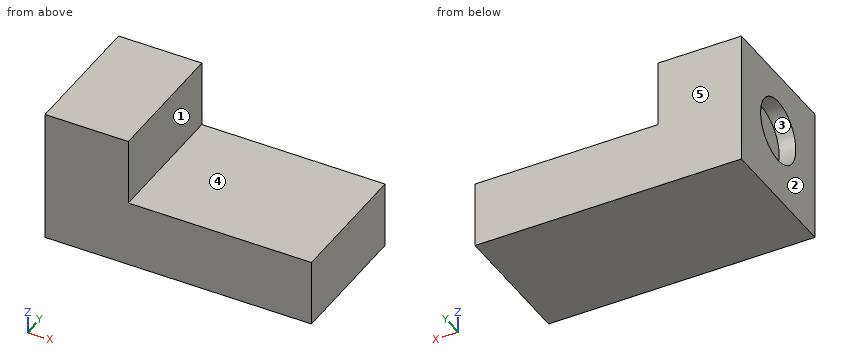
```python
from build123d import *

# Parameters (mm, degrees)
SKETCH_1_W          = 80
SKETCH_1_H          = 40
EXTRUDE_1_DEPTH     = 20
SKETCH_2_W          = 25
SKETCH_2_H          = 40
EXTRUDE_2_DEPTH     = 20
SKETCH_3_R          = 9.55930051
CUT_EXTRUDE_1_DEPTH = 5


with BuildPart() as part:
    # 草图1 → 凸台-拉伸1 (new body)
    with BuildSketch(Plane.XY):
        Rectangle(SKETCH_1_W, SKETCH_1_H)
    extrude(amount=EXTRUDE_1_DEPTH)

    # 草图2 → 凸台-拉伸2 (add)
    with BuildSketch(Plane.XY.offset(20)):
        with Locations((-27.5, 0)):
            Rectangle(SKETCH_2_W, SKETCH_2_H)
    extrude(amount=EXTRUDE_2_DEPTH)

    # 草图3 → 切除-拉伸1 (cut)
    with BuildSketch(Plane.ZY.offset(40)):
        with Locations((21.858234258, 0)):
            Circle(SKETCH_3_R)
    extrude(amount=-CUT_EXTRUDE_1_DEPTH, mode=Mode.SUBTRACT)


solid = part.part
```
Source: CAD feature listing. Evaluate the final solid. Frame: model axes, mm. Face numbers are marked on the shaded views. A direction names the side the tool comes from. Coordinates: 2 decimals unless noted, no trailing zeros. Loops run counter-clockwise (first coordinate to the right, second up) from the corner with the lowest first, then second, coordinate; pieces in that order, holes last. Notation, with made-up numbers: (33.5, 22.5) - (45.5, 22.5) arc R29 ccw to (45.5, 53.5) - close; hole circle Ø6 at (-17.5, -20.75). An arc over 180 degrees is marked (long way). Answer as CSV lines item,"result".
1. Section A-A (y = 0). Return loops of the section in (x, z), then the cut area to 3 significant figures.
Established:
outline,"(-40, 0) - (40, 0) - (40, 20) - (-15, 20) - (-15, 40) - (-40, 40) - (-40, 31.42) - (-35, 31.42) - (-35, 12.3) - (-40, 12.3) - close"
area,"2,000 mm2"
2. Section D-D (x = 25). Return loops of the section in (y, z), then the cut area to 3 significant figures.
Established:
outline,"(-20, 0) - (20, 0) - (20, 20) - (-20, 20) - close"
area,"800 mm2"
3. Mould query, pull axis Y, two halves, no side actions, for the marked faces 3, 4 and 5. Classes: released by +Y, released by -Y, zero draft, split by the parting line, or undercut.
Established:
face 3,"undercut"
face 4,"zero draft"
face 5,"released by +Y"
4. Reachability of the marked faces 1 and 2 from +Z, -Z, +X, -X, +Y, -Y: full face, straight path, thin tool, end or side. Return the list, or none.
Established:
face 1,"+Z, +X, +Y, -Y"
face 2,"+Z, -Z, -X, +Y, -Y"
5. Section B-B (z = 29.5). Return loops of the section in (x, y), then the cut area to 3 significant figures.
Established:
outline,"(-40, -20) - (-15, -20) - (-15, 20) - (-40, 20) - (-40, 5.74) - (-35, 5.74) - (-35, -5.74) - (-40, -5.74) - close"
area,"943 mm2"
6. Contact query for flat-ended pins moving along their axis: pin 1 (6 mm diameter, centred on y = -14, z = 29.5, fed in from +X); pin 2 (11.5 mm diameter, centred on y = 0, z = 21.86, fed in from -X). Output: stop coordinate, or through.
Established:
pin 1,"stops at x = -15"
pin 2,"stops at x = -35"
7. Section C-C (y = -11). Return loops of the section in (x, z).
Established:
outline,"(-40, 0) - (40, 0) - (40, 20) - (-15, 20) - (-15, 40) - (-40, 40) - close"
8. Ray query, line 1 (Z direction, x = 28.5, y = 17.5); line 2 (X direction, y = 4.5, z = 32.5); line 3 (X direction, y = 5, z = 15.5). Return the intervals inside material, ascending.
Established:
line 1,"z = 0 to 20"
line 2,"x = -40 to -15"
line 3,"x = -35 to 40"
